```python
from build123d import *

# Parameters (mm, degrees)
F0_R     = 18.45
F0_R_2   = 16.45
F1_DEPTH = 1.5
F2_R     = 0.25
F3_R     = 0.25
F4_R     = 0.25


with BuildPart() as f1:
    # F0 (on Front) → F1 (new body, symmetric)
    with BuildSketch(Plane.XZ):
        Circle(F0_R)
        Circle(F0_R_2, mode=Mode.SUBTRACT)
    extrude(amount=F1_DEPTH, both=True)

    # F2
    f2_edges = [f1.edges().sort_by_distance(p)[0] for p in [
        (-16.45, -1.5, 0),
    ]]
    fillet(f2_edges, radius=F2_R)

    # F3
    f3_edges = [f1.edges().sort_by_distance(p)[0] for p in [
        (-16.45, 1.5, 0),
    ]]
    fillet(f3_edges, radius=F3_R)

    # F4
    f4_edges = [f1.edges().sort_by_distance(p)[0] for p in [
        (-18.45, -1.5, 0),
        (-18.45, 1.5, 0),
    ]]
    fillet(f4_edges, radius=F4_R)


solid = f1.part
```
Verification items for the finished model (mm, model axes). Give positions to 0.01 mm unless a question says otherwise; leave off trailing zeros. Order: outer loops, then holes, each group sorted by start corner. A loop starts at its lowest first (then second) coordinate and runs counter-clockwise, first axis right, second up. Notation, with made-up numbers: M 56,22 L 109,22 A13 cw 109,41 Z; hole C -30.75,48.25 d2. An arc over 180 degrees is marked long. Answer in a Markdown table with one row per item. Add a question column.
Item 1: Scan lines: probe 1 along Z at (x, y) = (0, -0.45); probe 2 along X at (y, z) = (-0.7, -15); probe 3 along X at (y, z) = (1, -1.5). Record each from-to range of solid material in increasing order. Write a range as from..to.
Item 2: Section check C-C, the plane y = 0.2. Enter the section's corners in (x, z), and give its area (3 significant figures).
Item 3: Section check A-A, the plane z = 0. Enter the section's corners in (x, y).
Item 4: Section check B-B, the plane x = 0. Enter the section's corners in (y, z).
Item 5: Mould release check, pull along Y, two halves, no side actions. Record for faces 1 (the flat face through (8, -1.5, -15)), 2 (the cylindrical face through (-3.566, 0.018, -16.059)), 3 (the flat face through (8, 1.5, -15)): released by +Y, released by -Y, zero draft, split by the parting line, or undercut.
Item 6: Gauge pin test, flat ends, axial feed: pin 1 (8 mm diameter, centred on x = -10, z = -4.5, fed in from -Y); pin 2 (1 mm diameter, centred on x = 4.5, y = 1, fed in from +Z); pin 3 (1 mm diameter, centred on y = 0, z = 12, fed in from +X). Record the tip position at first contact, or that the pin passes through.
Filled sheet:
| question | item | result |
|---|---|---|
| 1 | probe 1 | z = -18.45..-16.45, 16.45..18.45 |
| 1 | probe 2 | x = -10.74..-6.75, 6.75..10.74 |
| 1 | probe 3 | x = -18.39..-16.38, 16.38..18.39 |
| 2 | outline | C 0,0 d36.9; hole C 0,0 d32.9 |
| 2 | area | 219 mm^2 |
| 3 | outline | M -18.45,-1.25 A0.25 ccw -18.2,-1.5 L -16.7,-1.5 A0.25 ccw -16.45,-1.25 L -16.45,1.25 A0.25 ccw -16.7,1.5 L -18.2,1.5 A0.25 ccw -18.45,1.25 Z; M 16.45,-1.25 A0.25 ccw 16.7,-1.5 L 18.2,-1.5 A0.25 ccw 18.45,-1.25 L 18.45,1.25 A0.25 ccw 18.2,1.5 L 16.7,1.5 A0.25 ccw 16.45,1.25 Z |
| 4 | outline | M -1.5,-18.2 A0.25 ccw -1.25,-18.45 L 1.25,-18.45 A0.25 ccw 1.5,-18.2 L 1.5,-16.7 A0.25 ccw 1.25,-16.45 L -1.25,-16.45 A0.25 ccw -1.5,-16.7 Z; M -1.5,16.7 A0.25 ccw -1.25,16.45 L 1.25,16.45 A0.25 ccw 1.5,16.7 L 1.5,18.2 A0.25 ccw 1.25,18.45 L -1.25,18.45 A0.25 ccw -1.5,18.2 Z |
| 5 | face 1 | released by -Y |
| 5 | face 2 | zero draft |
| 5 | face 3 | released by +Y |
| 6 | pin 1 | passes through |
| 6 | pin 2 | stops at z = 18.01 |
| 6 | pin 3 | stops at x = 14.43 |
